Input: part model. Units: mm. Frame: model coordinates. A direction names the side the tool comes from. Round coordinates to 2 decimals unless told otherwise and drop trailing zeros. Write each loop counter-clockwise with the first axis right and the second up, starting at its lowest first coordinate (ties: lowest second). Pieces come first, ordered by that corner, then holes. Notation, with made-up numbers: (72.25, 48) -> (117.25, 48) arc R29 cw to (117.25, 81) -> close; hole circle Ø5 at (50.25, 4). An arc over 180 degrees is marked (long way). Use CSV: the item, a comma, the result in double quotes.
```python
from build123d import *

# Parameters (mm, degrees)
CUT_EXTRUDE1_REACH      = 20.513
CUT_EXTRUDE1_END_RADIUS = 9.525
SKETCH2_R               = 1.9685


with BuildPart() as part:
    # Sketch1 → Revolve1 (revolve)
    with BuildSketch(Plane(origin=(0, 0, 0), x_dir=(0, 0, -1), z_dir=(1, 0, 0)), mode=Mode.PRIVATE) as revolve1_sk:
        Polygon((0, 3.175), (0, 6.35), (12.7, 6.35), (12.7, 9.525), (-12.7, 9.525), (-12.7, 3.175), align=None)
    revolve(revolve1_sk.sketch.rotate(Axis((0, 0, 0), (0, 0, 1)), 90), axis=Axis((0, 0, 0), (0, 0, 1)))

    # Cut-Extrude1: up to this cylinder (the profile starts inside it)
    cut_extrude1_end = Plane(origin=(0, 0, 0), z_dir=(0, 0, -1)) * Cylinder(CUT_EXTRUDE1_END_RADIUS, 73.776, mode=Mode.PRIVATE)
    # Sketch2 → Cut-Extrude1 (cut, up to the surface)
    with BuildSketch(Plane(origin=(0, 0, 0), x_dir=(1, 0, 0), z_dir=(0, 1, 0)), mode=Mode.PRIVATE) as cut_extrude1_sk1:
        with Locations(Location((0, -6.35, 0), (0, 0, 270))):
            Circle(SKETCH2_R)
    cut_extrude1_tool1 = extrude(cut_extrude1_sk1.sketch, amount=-CUT_EXTRUDE1_REACH, mode=Mode.PRIVATE) & cut_extrude1_end
    add(cut_extrude1_tool1.solids().sort_by_distance((0, 0, 6.35))[0], mode=Mode.SUBTRACT)
    # Sketch2 → Cut-Extrude1 (cut, up to the surface)
    with BuildSketch(Plane(origin=(0, 0, 0), x_dir=(1, 0, 0), z_dir=(0, 1, 0)), mode=Mode.PRIVATE) as cut_extrude1_sk2:
        with Locations(Location((0, 6.35, 0), (0, 0, 270))):
            Circle(SKETCH2_R)
    cut_extrude1_tool2 = extrude(cut_extrude1_sk2.sketch, amount=-CUT_EXTRUDE1_REACH, mode=Mode.PRIVATE) & cut_extrude1_end
    add(cut_extrude1_tool2.solids().sort_by_distance((0, 0, -6.35))[0], mode=Mode.SUBTRACT)


solid = part.part
```
Item 1: Section query C-C on z = -1. Return the cut outline in (x, y) (3 decimals).
Worked answers:
outline,"circle Ø19.05 at (0, 0); hole circle Ø12.7 at (0, 0)"
Item 2: Set-up query: faces 1 (the face through (0.69, 3.1, 6.26)), 2 (the face through (0.59, -7.76, -4.47)), 3 (the face through (-2.93, 5.634, -6.439)). Return all of +Z, -Z, +X, -X, +Y, -Y with unobstructed straight access to the full face (end or side cutting, diameter ignored); none if empty.
Worked answers:
face 1,"+Z, -Z"
face 2,"-Y"
face 3,"-Z"
Item 3: Pull-direction query (Y, two-part tool) for faces 4 (the face through (6.2, 2, -12.7)), 5 (the face through (2.06, 9.3, 0.18)), 6 (the face through (-2, -3, 0)); classes: +Y half, -Y half, draft (parallel to the pull), parting line (faces both ways), or undercut.
Worked answers:
face 4,"draft"
face 5,"parting line"
face 6,"undercut"
Item 4: Section query D-D on x = -5.75. Return the cut outline in (y, z), plus the area to 3 significant figures.
Worked answers:
outline,"(-7.59, -12.7) -> (-2.69, -12.7) -> (-2.69, 0) -> (2.69, 0) -> (2.69, -12.7) -> (7.59, -12.7) -> (7.59, 12.7) -> (-7.59, 12.7) -> close"
area,"317 mm²"
Item 5: First-contact query: pin 1 Ø5.5 at (x, y) = (0, 0) entering from -Z; pin 2 Ø3.5 at (x, z) = (0, 6.35) entering from -Y; pin 3 Ø5 at (x, z) = (-3, 7) entering from -Y. Flat tips, straight axial feed; report the tip coordinate or a pass-through.
Worked answers:
pin 1,"passes through"
pin 2,"stops at y = 2.65"
pin 3,"stops at y = -9.49"
Item 6: Section query A-A on y = 0. Return the cut outline in (x, z) (3 decimals), plus the area to 3 significant figures.
Worked answers:
outline,"(-9.525, -12.7) -> (-6.35, -12.7) -> (-6.35, 0) -> (-3.175, 0) -> (-3.175, 12.7) -> (-9.525, 12.7) -> close; (3.175, 0) -> (6.35, 0) -> (6.35, -12.7) -> (9.525, -12.7) -> (9.525, 12.7) -> (3.175, 12.7) -> close"
area,"242 mm²"
Item 7: Line query: line 1 (Z direction, x = 0, y = -4.75); line 2 (Z direction, x = 1.5, y = -7); line 3 (Y direction, x = 2, z = 9). Output: solid intervals per line, ascending.
Worked answers:
line 1,"z = 0 to 4.38, 8.32 to 12.7"
line 2,"z = -12.7 to -7.62, -5.08 to 5.08, 7.62 to 12.7"
line 3,"y = -9.31 to -2.47, 2.47 to 9.31"
Item 8: Section query B-B on x = 0. Give the number of separate pieces and of enclosed holes in the cut face, plus the area to 3 significant figures.
Worked answers:
separate pieces,"4"
enclosed holes,"0"
area,"204 mm²"
